from build123d import *

# Parameters (mm, degrees)
BOSS_EXTRUDE1_DEPTH = 15
SKETCH3_R           = 1.5
CUT_EXTRUDE1_DEPTH  = 2


with BuildPart() as part:
    # Sketch2 → Boss-Extrude1 (new body)
    with BuildSketch(Plane(origin=(0, 0, 0), x_dir=(0, 0, -1), z_dir=(1, 0, 0))):
        Polygon((0, 27), (10, 27), (10, 6.760833057), (30, 6.760833057), (30, 27), (165, 27), (165, 25), (32, 25), (32, 5), (8, 5), (8, 25), (2, 25), (2, 0), (0, 0), align=None)
    extrude(amount=BOSS_EXTRUDE1_DEPTH)

    # Sketch3 → Cut-Extrude1 (cut)
    with BuildSketch(Plane.XY):
        with Locations((7.5, 10)):
            Circle(SKETCH3_R)
    extrude(amount=-CUT_EXTRUDE1_DEPTH, mode=Mode.SUBTRACT)


solid = part.part
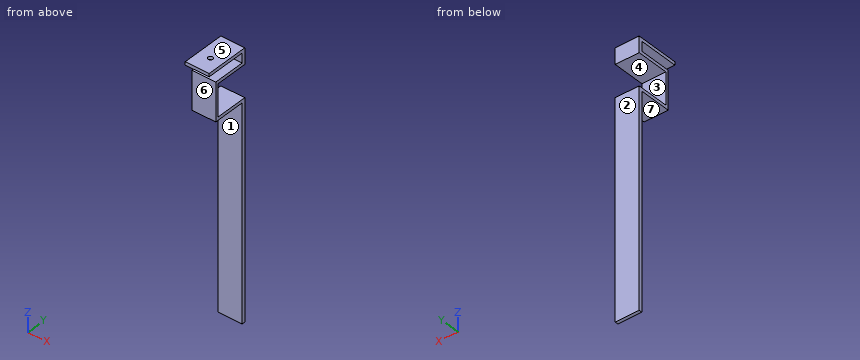
For this review, take the finished solid that the model builds, in its own axes (mm). Face numbers are marked on the shaded views. A direction names the side the tool comes from. Give positions to 0.01 mm unless a question says otherwise; leave off trailing zeros. Loops run counter-clockwise (first coordinate to the right, second up) from the corner with the lowest first, then second, coordinate; pieces in that order, holes last. Notation, with made-up numbers: (60, -0.5) -> (105, -0.5) arc R31 ccw to (105, 35.5) -> close; hole circle Ø6 at (52, 84). An arc over 180 degrees is marked (long way). One line per question, with ' | ' between items.
1) To check wall thickness, follow probe 1 along Z at (x, y) = (11.75, 12.5); probe 2 along Z at (x, y) = (14.5, 6.5); probe 3 along Y at (x, z) = (7.5, -1.55). State the ranges of each line that lie inside material, in increasing order.
Resolved:
probe 1: z = -32 to -30, -10 to -8, -2 to 0 | probe 2: z = -32 to -8, -2 to 0 | probe 3: y = 0 to 8.5, 11.5 to 27
2) We need section B-B (x = 7.5). Write out the cut boundary in (y, z), plus the area to 3 significant figures.
Resolved:
outline: (0, -2) -> (8.5, -2) -> (8.5, 0) -> (0, 0) -> close; (5, -32) -> (25, -32) -> (25, -165) -> (27, -165) -> (27, -30) -> (6.76, -30) -> (6.76, -10) -> (27, -10) -> (27, 0) -> (11.5, 0) -> (11.5, -2) -> (25, -2) -> (25, -8) -> (5, -8) -> close | area: 449 mm2
3) We need section A-A (y = 10). Write out the cut boundary in (x, z).
Resolved:
outline: (0, -32) -> (15, -32) -> (15, -30) -> (0, -30) -> close; (0, -10) -> (15, -10) -> (15, -8) -> (0, -8) -> close; (0, -2) -> (6, -2) -> (6, 0) -> (0, 0) -> close; (9, -2) -> (15, -2) -> (15, 0) -> (9, 0) -> close
4) We need section C-C (z = -73.5). Write out the cut boundary in (x, y), plus the area to 3 significant figures.
Resolved:
outline: (0, 25) -> (15, 25) -> (15, 27) -> (0, 27) -> close | area: 30.0 mm2
5) The part is to be moulded in two halves that separate along Z. For the marked faces 4, 5, 6 and 7, say which applies: +Z half, -Z half, draft (parallel to the pull), parting line (faces both ways), or undercut.
Resolved:
face 4: undercut | face 5: +Z half | face 6: draft | face 7: -Z half
6) For the marked faces 1, 2 and 3, list the 3-axis set-ups (+Z, -Z, +X, -X, +Y, -Y) from which the entire face can be reached by the end or side of a thin tool; tool diameter is ignored.
Resolved:
face 1: -Z, +X, -X, -Y | face 2: +Z, -Z, +X, -X, +Y | face 3: +X, -X, +Y
7) Insertion check: pin 1 Ø5 at (x, y) = (7.5, 10) entering from +Z; pin 2 Ø1.5 at (x, z) = (7.5, -47) entering from -Y. Each pin has a flat end and moves straight along its axis. Give the tip position at first contact, or say it passes through.
Resolved:
pin 1: stops at z = 0 | pin 2: stops at y = 25
